Read the model definition and answer for the solid it produces. Units are mm, in the model's axes. Round coordinates to 2 decimals unless told otherwise and drop trailing zeros. Order: outer loops, then holes, each group sorted by start corner. A loop starts at its lowest first (then second) coordinate and runs counter-clockwise, first axis right, second up.
from build123d import *

# Parameters (mm, degrees)
EXTRUDE_1_DEPTH              = 8
HOLE_WIZARD_M4_1_D           = 3.3
HOLE_WIZARD_M4_1_CSINK_D     = 4.05
HOLE_WIZARD_M4_1_CSINK_ANGLE = 90


with BuildPart() as part:
    # 草图1 → 凸台-拉伸1 (new body)
    with BuildSketch(Plane.XY):
        Polygon((3.464101615, 0), (1.732050808, 3), (-1.732050808, 3), (-3.464101615, 0), (-1.732050808, -3), (1.732050808, -3), align=None)
    extrude(amount=EXTRUDE_1_DEPTH)

    # M4 螺纹孔1 (through all)
    with Locations(Plane(origin=(0, 0, 0), x_dir=(-1, 0, 0), z_dir=(0, 0, -1))):
        with Locations((0, 0)):
            CounterSinkHole(HOLE_WIZARD_M4_1_D / 2, HOLE_WIZARD_M4_1_CSINK_D / 2, counter_sink_angle=HOLE_WIZARD_M4_1_CSINK_ANGLE)


solid = part.part
Q1. A cutting plane is placed at C-C, the plane y = -2.5. Give the vertices of the cut face in (x, z).
Outcome:
outline: (-2.02, 0) - (2.02, 0) - (2.02, 8) - (-2.02, 8) - close
Q2. A cutting plane is placed at D-D, the plane x = -2.5. Give the vertices of the cut face in (y, z), plus the area to 3 significant figures.
Outcome:
outline: (-1.67, 0) - (1.67, 0) - (1.67, 8) - (-1.67, 8) - close
area: 26.7 mm2
Q3. For a pull along Y with two mould halves and no side action, classify faces 1 (the face through (0, 3, 4)), 2 (the face through (-2.6, -1.5, 3.9)), 3 (the face through (1.5, 1.4, 8)), 4 (the face through (-1.216, 1.115, 4.241)) as released by +Y, released by -Y, zero draft, split by the parting line, or undercut.
Outcome:
face 1: released by +Y
face 2: released by -Y
face 3: zero draft
face 4: undercut
Q4. A cutting plane is placed at A-A, the plane x = 0. Give the vertices of the cut face in (y, z) (3 decimals), plus the area to 3 significant figures.
Outcome:
outline: (-3, 0) - (-2.025, 0) - (-1.65, 0.375) - (-1.65, 8) - (-3, 8) - close; (1.65, 0.375) - (2.025, 0) - (3, 0) - (3, 8) - (1.65, 8) - close
area: 21.5 mm2
Q5. Straight lines are drawn through the part: probe 1 along Y at (x, z) = (0, 0.5); probe 2 along X at (y, z) = (0.5, 6); probe 3 along X at (y, z) = (1.5, 6.25). For each, find the intervals that lie inside material, in ascending order.
Outcome:
probe 1: y = -3 to -1.65, 1.65 to 3
probe 2: x = -3.18 to -1.57, 1.57 to 3.18
probe 3: x = -2.6 to -0.69, 0.69 to 2.6
Q6. Flat-ended cylindrical pins translate along their axes: pin 1 (3 mm diameter, centred on x = 0, y = 0, fed in from +Z) (1 decimal); pin 2 (2 mm diameter, centred on y = 1.5, z = 4, fed in from -X). Find the tip coordinate at first contact, or state that the pin passes through.
Outcome:
pin 1: passes through
pin 2: stops at x = -3.18
Q7. A cutting plane is placed at B-B, the plane z = 6.75. Give the vertices of the cut face in (x, y), plus the area to 3 significant figures.
Outcome:
outline: (-3.46, 0) - (-1.73, -3) - (1.73, -3) - (3.46, 0) - (1.73, 3) - (-1.73, 3) - close; hole circle Ø3.3 at (0, 0)
area: 22.6 mm2
